Work out the finished part from the listing and answer in its coordinate system (mm). A direction names the side the tool comes from. Coordinates: 2 decimals unless noted, no trailing zeros. Write each loop counter-clockwise with the first axis right and the second up, starting at its lowest first coordinate (ties: lowest second). Pieces come first, ordered by that corner, then holes. Notation, with made-up numbers: (58, 64) - (114, 64) arc R23 ccw to (114, 99) - close; hole circle Ø4 at (-25.5, 73.25). An arc over 180 degrees is marked (long way). Use one line per item in the form item = value. Start each with the question number.
Item 1: A cutting plane is placed at D-D (z = 25.5). Write down the section's boundary in (x, y).
Item 2: Consider probe 1 along Y at (x, z) = (30.5, 18.5); probe 2 along X at (y, z) = (-20.5, 16); probe 3 along X at (y, z) = (-41, 10). Determine where each line is inside the solid, lowest interval first.
Item 3: For faces 1 (the cylindrical face through (23.822, -37.873, 7.315)), 2 (the flat face through (25, 25, 30)), determine the directions among +Z, -Z, +X, -X, +Y, -Y from which every point of the face is accessible in a straight line to the end or side of a thin tool.
Item 4: A cutting plane is placed at A-A (z = 17). Write down the section's boundary in (x, y).
Item 5: A cutting plane is placed at C-C (x = 32.5). Write down the section's boundary in (y, z).
Item 6: A cutting plane is placed at B-B (x = 15). Write down the section's boundary in (y, z), then the cut area to 3 significant figures.
from build123d import *

# Parameters (mm, degrees)
F1_W     = 50
F1_H     = 30
F2_DEPTH = 50
F3_R     = 7.2976744804
F4_DEPTH = 76.8214575
F5_DEPTH = 116.5


# Not quite as in the source:
# - an extrude ends at something that could not be found from the text; its depth is read off the source's solid


with BuildPart() as f2:
    # F1 (on Right) → F2 (new body)
    with BuildSketch(Plane.YZ):
        with Locations((25, 15)):
            Rectangle(F1_W, F1_H)
    extrude(amount=F2_DEPTH)

    # F3 (on face) → F4 (join, through all)
    with BuildSketch(Plane.XZ):
        with Locations((20.4548016191, 13.7891862541)):
            Circle(F3_R)
    extrude(amount=F4_DEPTH)

    # F5 (add): a face of the model
    f5_faces = [f2.faces().sort_by_distance(p)[0] for p in [
        (20.4548016191, -76.8214575, 13.7891862541),
    ]]
    extrude(f5_faces, amount=-F5_DEPTH)


solid = f2.part
Answer:
q1.outline = (0, 0) - (50, 0) - (50, 50) - (0, 50) - close
q2.probe_1 = 0 to 50
q2.probe_2 = 13.5 to 27.41
q2.probe_3 = 14.22 to 26.69
q3.face_1 = -Y
q3.face_2 = +Z, +X, -X, +Y, -Y
q4.outline = (0, 0) - (13.9, 0) - (13.9, -76.82) - (27.01, -76.82) - (27.01, 0) - (50, 0) - (50, 50) - (0, 50) - close
q5.outline = (0, 0) - (50, 0) - (50, 30) - (0, 30) - close
q6.outline = (-76.82, 8.94) - (0, 8.94) - (0, 0) - (50, 0) - (50, 30) - (0, 30) - (0, 18.64) - (-76.82, 18.64) - close
q6.area = 2,240 mm²
